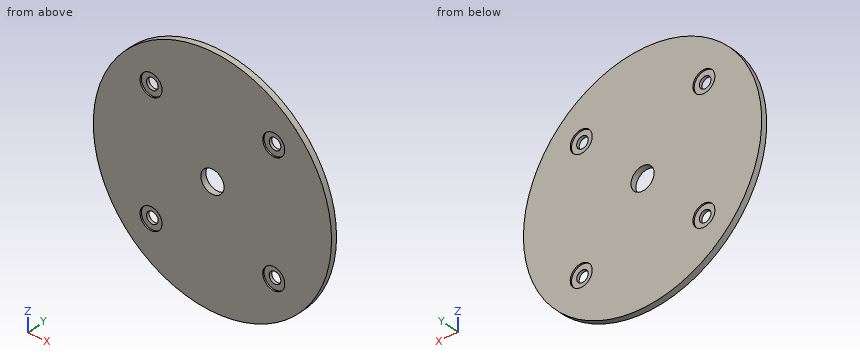
```python
from build123d import *

# Parameters (mm, degrees)
SKETCH2_R                   = 65.405
BOSS_EXTRUDE1_DEPTH         = 1.5875
F_1_4_0_25_DIAMETER_HOLE1_D = 6.35
F_1_2_0_5_DIAMETER_HOLE1_D  = 12.7
SKETCH10_R                  = 6.0325
CUT_EXTRUDE1_DEPTH          = 0.79375


with BuildPart() as part:
    # Sketch2 → Boss-Extrude1 (new body, symmetric)
    with BuildSketch(Plane(origin=(0, 0, 0), x_dir=(1, 0, 0), z_dir=(0, 1, 0))):
        Circle(SKETCH2_R)
    extrude(amount=BOSS_EXTRUDE1_DEPTH, both=True)

    # 1/4 (0.25) Diameter Hole1 (through all)
    with Locations(Plane(origin=(0, 1.5875, 0), x_dir=(1, 0, 0), z_dir=(0, 1, 0))):
        with Locations((-33.675960454, -33.675960454), (-33.675960454, 33.675960454), (33.675960454, 33.675960454), (33.675960454, -33.675960454)):
            Hole(F_1_4_0_25_DIAMETER_HOLE1_D / 2)

    # 1/2 (0.5) Diameter Hole1 (through all)
    with Locations(Plane(origin=(0, 1.5875, 0), x_dir=(1, 0, 0), z_dir=(0, 1, 0))):
        with Locations((0, 0)):
            Hole(F_1_2_0_5_DIAMETER_HOLE1_D / 2)

    # Sketch10 → Cut-Extrude1 (cut)
    with BuildSketch(Plane(origin=(0, 1.5875, 0), x_dir=(1, 0, 0), z_dir=(0, 1, 0))):
        with Locations((-33.675960454, 33.675960454)):
            Circle(SKETCH10_R)
        with Locations((33.675960454, 33.675960454)):
            Circle(SKETCH10_R)
        with Locations((33.675960454, -33.675960454)):
            Circle(SKETCH10_R)
        with Locations((-33.675960454, -33.675960454)):
            Circle(SKETCH10_R)
    cut_extrude1 = extrude(amount=-CUT_EXTRUDE1_DEPTH, mode=Mode.SUBTRACT)

    # Mirror1: Cut-Extrude1 across plane
    add(cut_extrude1.mirror(Plane.ZX), mode=Mode.SUBTRACT)


solid = part.part
```
Input: part model. Units: mm. Frame: model coordinates. Give positions to 0.01 mm unless a question says otherwise; leave off trailing zeros. Loops run counter-clockwise (first coordinate to the right, second up) from the corner with the lowest first, then second, coordinate; pieces in that order, holes last.
1) Line query: L1, parallel to Z at x = -31, y = -1.1; L2, parallel to Z at x = 32.5, y = -0.1; L3, parallel to X at y = -0.3, z = -35. Output: solid intervals per line, ascending.
A:
L1: z = -57.59 to -39.08, -28.27 to 28.27, 39.08 to 57.59
L2: z = -56.76 to -36.63, -30.73 to 30.73, 36.63 to 56.76
L3: x = -55.25 to -36.56, -30.79 to 30.79, 36.56 to 55.25
2) Contact query for flat-ended pins moving along their axis: pin 1 (15.5 mm diameter, centred on x = -33.68, z = -33.68, fed in from +Y); pin 2 (1.5 mm diameter, centred on x = -18.5, y = 0.5, fed in from -Z); pin 3 (3.5 mm diameter, centred on x = -35.5, z = 35.5, fed in from -Y); pin 4 (1.5 mm diameter, centred on y = -0.5, z = -32, fed in from -X). Output: stop coordinate, or through.
A:
pin 1: stops at y = 1.59
pin 2: stops at z = -62.95
pin 3: stops at y = -0.79
pin 4: stops at x = -57.46
3) Section query D-D on z = -24. Return the cut outline in (x, y), and give its area (3 significant figures).
A:
outline: (-60.84, -1.59) - (60.84, -1.59) - (60.84, 1.59) - (-60.84, 1.59) - close
area: 386 mm2
4) Section query C-C on y = -0.3. Return the cut outline in (x, z) (3 decimals), and give its area (3 significant figures).
A:
outline: circle Ø130.81 at (0, 0); hole circle Ø6.35 at (-33.676, -33.676); hole circle Ø6.35 at (-33.676, 33.676); hole circle Ø12.7 at (0, 0); hole circle Ø6.35 at (33.676, -33.676); hole circle Ø6.35 at (33.676, 33.676)
area: 13,200 mm2
